```python
from build123d import *

# Parameters (mm, degrees)
ESQUISSE1_R               = 3
T_LE_DE_BASE_PLI_E1_DEPTH = 0.7366


# Sheet-metal steps are written as plain solids
with BuildPart() as part:
    # Esquisse1 → Tôle de base pliée1 (new body)
    with BuildSketch(Plane.XY):
        with BuildLine():
            Line((32.6051263, -9.780978848), (59.980728888, -3.900810235))
            ThreePointArc((59.980728888, -3.900810235), (63.060247102, -0.788250523), (61.443305942, 3.280774136))
            Line((61.443305942, 3.280774136), (30.370857933, 25.155484984))
            ThreePointArc((30.370857933, 25.155484984), (25.994902612, 25.305403023), (24.103274011, 21.356580209))
            Line((24.103274011, 21.356580209), (27.800119432, -6.398299253))
            ThreePointArc((27.800119432, -6.398299253), (29.46250107, -9.14096248), (32.6051263, -9.780978848))
        make_face()
        with Locations((28.068256791, 21.884700983)):
            Circle(ESQUISSE1_R, mode=Mode.SUBTRACT)
        with Locations((31.765102212, -5.870178479)):
            Circle(ESQUISSE1_R, mode=Mode.SUBTRACT)
        with Locations((59.1407048, 0.009990135)):
            Circle(ESQUISSE1_R, mode=Mode.SUBTRACT)
    extrude(amount=-T_LE_DE_BASE_PLI_E1_DEPTH)


solid = part.part
```
Read the model definition and answer for the solid it produces. Units are mm, in the model's axes. Give positions to 0.01 mm unless a question says otherwise; leave off trailing zeros. Loops run counter-clockwise (first coordinate to the right, second up) from the corner with the lowest first, then second, coordinate; pieces in that order, holes last.
Item 1: The part is cut by section A-A (x = 31.5). Write down the section's boundary in (y, z).
Item 2: The part is cut by section D-D (x = 41.5). Write down the section's boundary in (y, z).
Item 3: This flat-tipped pin is pushed along its axis until it touches: pin 1 Ø5.5 at (x, y) = (59.14, 0.01) entering from +Z. Where does it stop, or does it pass through?
Item 4: Find the intervals of material crossed by line 1 along Y through (x, z) = (30.5, -0.1); line 2 along Y through (x, z) = (31.5, -0.1); line 3 along Y through (x, z) = (61, -0.2), in increasing order.
Item 5: The part is cut by section C-C (z = -0.5). Write down the section's boundary in (x, y), and give its area (3 significant figures).
Item 6: The mould has two halves that part along Y. Classify faces 1 (the cylindrical face through (63.047, -0.852, -0.363)), 2 (the flat face through (39, 4, 0)), 3 (the cylindrical face through (29.42, -9.11, -0.36)), 4 (the cylindrical face through (56.144, 0.142, -0.363)): released by +Y, released by -Y, zero draft, split by the parting line, or undercut.
Item 7: The part is cut by section B-B (y = -7.5). Write down the section's boundary in (x, z).
Taken from the geometry:
1. outline: (-9.86, -0.74) - (-8.86, -0.74) - (-8.86, 0) - (-9.86, 0) - close; (-2.88, -0.74) - (24.36, -0.74) - (24.36, 0) - (-2.88, 0) - close
2. outline: (-7.87, -0.74) - (17.32, -0.74) - (17.32, 0) - (-7.87, 0) - close
3. pin 1: passes through
4. line 1: y = -9.66 to -8.59, -3.15 to 20.13, 23.64 to 25.06
4. line 2: y = -9.86 to -8.86, -2.88 to 24.36
4. line 3: y = -3.53 to -2.34, 2.36 to 3.59
5. outline: (24.1, 21.36) - (27.8, -6.4) arc R4 ccw to (32.61, -9.78) - (59.98, -3.9) arc R4 ccw to (61.44, 3.28) - (30.37, 25.16) arc R4 ccw to start; hole circle Ø6 at (28.07, 21.88); hole circle Ø6 at (31.77, -5.87); hole circle Ø6 at (59.14, 0.01)
5. area: 732 mm2
6. face 1: split by the parting line
6. face 2: zero draft
6. face 3: released by -Y
6. face 4: undercut
7. outline: (28.11, -0.74) - (29.25, -0.74) - (29.25, 0) - (28.11, 0) - close; (34.28, -0.74) - (43.22, -0.74) - (43.22, 0) - (34.28, 0) - close
